Could you check a few things on this model? Use its own coordinates, in mm. Face numbers are marked on the shaded views. A direction names the side the tool comes from. Give positions to 0.01 mm unless a question says otherwise; leave off trailing zeros. Write each loop counter-clockwise with the first axis right and the second up, starting at its lowest first coordinate (ties: lowest second). Pieces come first, ordered by that corner, then holes. Notation, with made-up numbers: (-4, -15) -> (15, -15) arc R26 cw to (15, 7) -> close; hole circle Ø1 at (44.25, 69.25). An arc over 180 degrees is marked (long way). One line per question, with ' | ' between items.
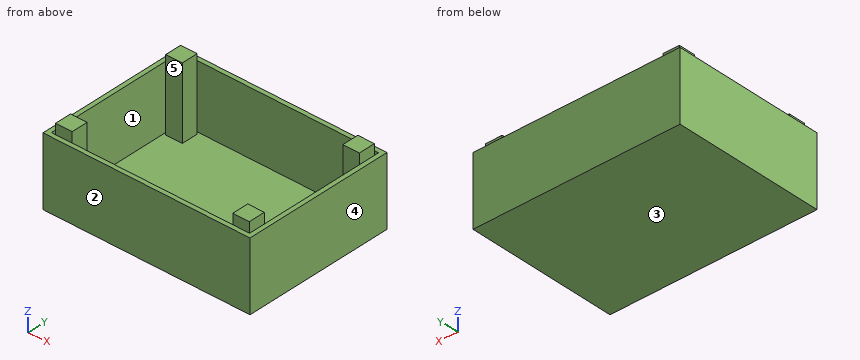
from build123d import *

# Parameters (mm, degrees)
F0_W     = 6
F0_H     = 6
F1_DEPTH = 28
F0_W_2   = 75
F0_H_2   = 55
F2_DEPTH = 25
F3_DEPTH = 1.8


with BuildPart() as f1:
    # F0 (on Top) → F1 (new body)
    with BuildSketch(Plane.XY):
        with Locations((-32.1, 22.1)):
            Rectangle(F0_W, F0_H)
    extrude(amount=F1_DEPTH)



with BuildPart() as f1b:
    # F0 (on Top) → F1, piece 2 (new body)
    with BuildSketch(Plane.XY):
        with Locations((32.1, 22.1)):
            Rectangle(F0_W, F0_H)
    extrude(amount=F1_DEPTH)


with BuildPart() as f1c:
    # F0 (on Top) → F1, piece 3 (new body)
    with BuildSketch(Plane.XY):
        with Locations((-32.1, -22.1)):
            Rectangle(F0_W, F0_H)
    extrude(amount=F1_DEPTH)


with BuildPart() as f1d:
    # F0 (on Top) → F1, piece 4 (new body)
    with BuildSketch(Plane.XY):
        with Locations((32.1, -22.1)):
            Rectangle(F0_W, F0_H)
    extrude(amount=F1_DEPTH)


with BuildPart() as f2:
    # F0 (on Top) → F2 (new body)
    with BuildSketch(Plane.XY):
        Rectangle(F0_W_2, F0_H_2)
        Polygon((-35.9, 25.1), (-35.9, 25.9), (-35.1, 25.9), (35.1, 25.9), (35.9, 25.9), (35.9, 25.1), (35.9, -25.1), (35.9, -25.9), (35.1, -25.9), (-35.1, -25.9), (-35.9, -25.9), (-35.9, -25.1), align=None, mode=Mode.SUBTRACT)
    extrude(amount=F2_DEPTH)


with BuildPart() as f1_1:
    add(f1.part)

    add(f1b.part)  # F3 merges F1b

    add(f1c.part)  # F3 merges F1c

    add(f1d.part)  # F3 merges F1d

    add(f2.part)  # F3 merges F2
    # F0 (on Top) → F3 (join)
    with BuildSketch(Plane.XY):
        Polygon((-35.1, 25.9), (-35.9, 25.9), (-35.9, 25.1), (-35.9, -25.1), (-35.9, -25.9), (-35.1, -25.9), (35.1, -25.9), (35.9, -25.9), (35.9, -25.1), (35.9, 25.1), (35.9, 25.9), (35.1, 25.9), align=None)
        with Locations((-32.1, -22.1)):
            Rectangle(F0_W, F0_H, mode=Mode.SUBTRACT)
        with Locations((32.1, -22.1)):
            Rectangle(F0_W, F0_H, mode=Mode.SUBTRACT)
        with Locations((-32.1, 22.1)):
            Rectangle(F0_W, F0_H, mode=Mode.SUBTRACT)
        with Locations((32.1, 22.1)):
            Rectangle(F0_W, F0_H, mode=Mode.SUBTRACT)
    extrude(amount=F3_DEPTH)


solid = f1_1.part
Q1. Will these pins go through, and if not, where does the flat tip stop? pin 1 (1.5 mm diameter, centred on x = -26, y = 12.5, fed in from +Z); pin 2 (6 mm diameter, centred on x = 22, y = 14.5, fed in from -Z).
Answer below:
pin 1: stops at z = 1.8 | pin 2: stops at z = 0
Q2. On a 3-axis mill with a long thin cutter (end or side, diameter ignored), from which of +Z, -Z, +X, -X, +Y, -Y can I reach the whole of each face in a straight line? I mean the marked faces 1 and 2. Say none if no direction works.
Answer below:
face 1: +Z | face 2: +Z, -Z, +X, -X, -Y
Q3. Imagine slicing it at A-A on z = 13. Please give me the cut outline in (x, y).
Answer below:
outline: (-37.5, -27.5) -> (37.5, -27.5) -> (37.5, 27.5) -> (-37.5, 27.5) -> close; (-35.1, -25.1) -> (-29.1, -25.1) -> (-29.1, -19.1) -> (-35.1, -19.1) -> close; (-35.1, 19.1) -> (-29.1, 19.1) -> (-29.1, 25.1) -> (-35.1, 25.1) -> close; (29.1, -25.1) -> (35.1, -25.1) -> (35.1, -19.1) -> (29.1, -19.1) -> close; (29.1, 19.1) -> (35.1, 19.1) -> (35.1, 25.1) -> (29.1, 25.1) -> close; hole (-35.9, -25.9) -> (35.9, -25.9) -> (35.9, 25.9) -> (-35.9, 25.9) -> close
Q4. If we mould it in two halves opening along X, with no side actions, what happens to the marked faces 3, 4 and 5? For each: +X half, -X half, draft (parallel to the pull), parting line (faces both ways), or undercut.
Answer below:
face 3: draft | face 4: +X half | face 5: undercut
Q5. If I drill on line 1 along Y through (x, z) = (-33, 16.5); line 2 along Y through (x, z) = (-15, 19.5); line 3 along X through (y, z) = (-16, 8), over which ranges is the centre line in solid material (lowest first)?
Answer below:
line 1: y = -27.5 to -25.9, -25.1 to -19.1, 19.1 to 25.1, 25.9 to 27.5 | line 2: y = -27.5 to -25.9, 25.9 to 27.5 | line 3: x = -37.5 to -35.9, 35.9 to 37.5
Q6. Imagine slicing it at B-B on y = 17.5. Please give me the cut outline in (x, z).
Answer below:
outline: (-37.5, 0) -> (37.5, 0) -> (37.5, 25) -> (35.9, 25) -> (35.9, 1.8) -> (-35.9, 1.8) -> (-35.9, 25) -> (-37.5, 25) -> close
Q7. Imagine slicing it at C-C on x = -23. Please give me the cut outline in (y, z), and give its area (3 significant figures).
Answer below:
outline: (-27.5, 0) -> (27.5, 0) -> (27.5, 25) -> (25.9, 25) -> (25.9, 1.8) -> (-25.9, 1.8) -> (-25.9, 25) -> (-27.5, 25) -> close | area: 173 mm^2
Q8. Imagine slicing it at D-D on x = 32. Please give me the cut outline in (y, z).
Answer below:
outline: (-27.5, 0) -> (27.5, 0) -> (27.5, 25) -> (25.9, 25) -> (25.9, 1.8) -> (25.1, 1.8) -> (25.1, 28) -> (19.1, 28) -> (19.1, 1.8) -> (-19.1, 1.8) -> (-19.1, 28) -> (-25.1, 28) -> (-25.1, 1.8) -> (-25.9, 1.8) -> (-25.9, 25) -> (-27.5, 25) -> close
